Work out the finished part from the listing and answer in its coordinate system (mm). Face numbers are marked on the shaded views. A direction names the side the tool comes from. Coordinates: 2 decimals unless noted, no trailing zeros. Order: outer loops, then holes, each group sorted by start corner. A loop starts at its lowest first (then second) coordinate and runs counter-clockwise, first axis right, second up. Notation, with made-up numbers: M 47,85 L 67,85 A26 cw 67,115 Z; hole C -20.75,16 d3. An arc over 180 degrees is marked long. Write item = value, one per line. Start each with the question number.
Q1. Each of these flat-tipped pins is pushed along its axis until it touches: P1, Ø6, axis at x = -9.5, y = -1.5, coming from the +Z side; P2, Ø12, axis at x = -5, y = -5, coming from the -Z side; P3, Ø4.5, axis at x = 3.75, y = 0, coming from the +Z side; P4, Ø4, axis at x = -3.75, y = 0, coming from the +Z side. Where does it stop, or does it pass through?
Q2. Straight lines are drawn through the part: line 1 along Y through (x, z) = (-25, 1.55); line 2 along Y through (x, z) = (-14.5, 6.25); line 3 along Z through (x, y) = (-6.5, 3.75). For each, find the intervals that lie inside material, in ascending order.
Q3. Find section C-C on z = 3.5. Give the vertices of the cut face in (x, y).
Q4. A tool of negligible diameter and unlimited length cuts with its end or side. For the marked faces 4 and 5, from which of +Z, -Z, +X, -X, +Y, -Y can it reach the whole face along a straight path? Write none if from no direction.
Q5. Determine the mould class of the marked faces 1, 2 and 3 for opening direction Y: released by +Y, released by -Y, zero draft, split by the parting line, or undercut.
Q6. Find section A-A on y = 0. Give the vertices of the cut face in (x, z).
Q7. Find section D-D on x = 15. Give the vertices of the cut face in (y, z).
Q8. Find section B-B on x = -3.75. Give the vertices of the cut face in (y, z).
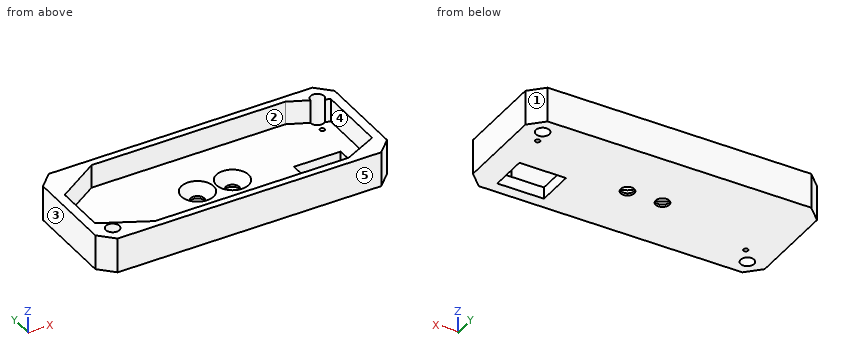
```python
from build123d import *

# Parameters (mm, degrees)
SKETCH_1_W          = 62.5
SKETCH_1_H          = 25
EXTRUDE_1_DEPTH     = 2.5
SKETCH_2_R          = 1.45
CUT_EXTRUDE_1_DEPTH = 3.5
CHAMFER_1_SIZE      = 2
SKETCH_3_W          = 62.5
SKETCH_3_H          = 25
EXTRUDE_2_DEPTH     = 5
SKETCH_4_W          = 10
SKETCH_4_H          = 8
CUT_EXTRUDE_2_DEPTH = 5
SKETCH_5_W          = 67.566121691
SKETCH_5_H          = 29.988395665
CUT_EXTRUDE_3_DEPTH = 10
SKETCH_7_R          = 1.45
CUT_EXTRUDE_4_DEPTH = 10
SKETCH_10_R         = 0.5
CUT_EXTRUDE_5_DEPTH = 10


with BuildPart() as part:
    # Эскиз1 → Бобышка-Вытянуть1 (new body)
    with BuildSketch(Plane.XY):
        Rectangle(SKETCH_1_W, SKETCH_1_H)
    extrude(amount=EXTRUDE_1_DEPTH)

    # Эскиз2 → Вырез-Вытянуть1 (cut)
    with BuildSketch(Plane.XY.offset(2.5)):
        with Locations((3.75, 0)):
            Circle(SKETCH_2_R)
        with Locations((-3.75, 0)):
            Circle(SKETCH_2_R)
    extrude(amount=-CUT_EXTRUDE_1_DEPTH, mode=Mode.SUBTRACT)

    # Фаска1
    chamfer_1_edges = [part.edges().sort_by_distance(p)[0] for p in [
        (2.3, 0, 2.5),
        (-5.2, 0, 2.5),
    ]]
    chamfer(chamfer_1_edges, length=CHAMFER_1_SIZE)

    # Эскиз3 → Бобышка-Вытянуть2 (add)
    with BuildSketch(Plane.XY.offset(2.5)):
        Rectangle(SKETCH_3_W, SKETCH_3_H)
        Polygon((-29.25, -6), (-29.25, 5), (-19.95, 11), (21.55, 11), (29.25, 7.5), (29.25, -7.5), (22.14795897, -11), (-19.35204103, -11), align=None, mode=Mode.SUBTRACT)
    extrude(amount=EXTRUDE_2_DEPTH)

    # Эскиз4 → Вырез-Вытянуть2 (cut)
    with BuildSketch(Plane(origin=(0, 0, 0), x_dir=(-1, 0, 0), z_dir=(0, 0, -1))):
        with Locations((-20.75, -6)):
            Rectangle(SKETCH_4_W, SKETCH_4_H)
    extrude(amount=-CUT_EXTRUDE_2_DEPTH, mode=Mode.SUBTRACT)

    # Эскиз5 → Вырез-Вытянуть3 (cut)
    with BuildSketch(Plane.XY.offset(7.5)):
        with Locations((0.466014855, 0.289583976)):
            Rectangle(SKETCH_5_W, SKETCH_5_H)
        Polygon((-28.25, 12.5), (-31.25, 9.5), (-31.25, -9.5), (-28.25, -12.5), (28.25, -12.5), (31.25, -9.5), (31.25, 9.5), (28.25, 12.5), align=None, mode=Mode.SUBTRACT)
    extrude(amount=-CUT_EXTRUDE_3_DEPTH, mode=Mode.SUBTRACT)

    # Эскиз7 → Вырез-Вытянуть4 (cut)
    with BuildSketch(Plane.XY.offset(7.5)):
        with Locations((-27.25, -9)):
            Circle(SKETCH_7_R)
        with Locations(Location((27.25, 9, 0), (0, 0, 313.779004768))):
            Circle(SKETCH_7_R)
    extrude(amount=-CUT_EXTRUDE_4_DEPTH, mode=Mode.SUBTRACT)

    # Эскиз10 → Вырез-Вытянуть5 (cut)
    with BuildSketch(Plane.XY.offset(2.5)):
        with Locations((-25, -5.766085635)):
            Circle(SKETCH_10_R)
        with Locations((26.547958971, 6)):
            Circle(SKETCH_10_R)
    extrude(amount=-CUT_EXTRUDE_5_DEPTH, mode=Mode.SUBTRACT)


solid = part.part
```
Findings below:
q1.P1 = 2.5
q1.P2 = 0
q1.P3 = 1.3
q1.P4 = 1.05
q2.line_1 = -12.5 to -6.27, -5.27 to 12.5
q2.line_2 = -12.5 to -11, 11 to 12.5
q2.line_3 = 0 to 2.5
q3.outline = M -31.25,-9.5 L -28.25,-12.5 L 28.25,-12.5 L 31.25,-9.5 L 31.25,9.5 L 28.25,12.5 L -28.25,12.5 L -31.25,9.5 Z; hole M -29.25,-6 L -19.35,-11 L 22.15,-11 L 24.18,-10 L 25.75,-10 L 25.75,-9.22 L 29.25,-7.5 L 29.25,7.5 L 28.25,7.95 A1.45 ccw long 25.8,9.07 L 21.55,11 L -19.95,11 L -29.25,5 Z; hole C -27.25,-9 d2.9
q4.face_4 = +Z
q4.face_5 = +Z, -Z, +X, -X, -Y
q5.face_1 = released by +Y
q5.face_2 = undercut
q5.face_3 = zero draft
q6.outline = M -31.25,0 L -5.2,0 L -5.2,0.5 L -7.2,2.5 L -29.25,2.5 L -29.25,7.5 L -31.25,7.5 Z; M -2.3,0 L 2.3,0 L 2.3,0.5 L 0.3,2.5 L -0.3,2.5 L -2.3,0.5 Z; M 5.2,0 L 31.25,0 L 31.25,7.5 L 29.25,7.5 L 29.25,2.5 L 7.2,2.5 L 5.2,0.5 Z
q7.outline = M -12.5,0 L 12.5,0 L 12.5,7.5 L 11,7.5 L 11,2.5 L -11,2.5 L -11,7.5 L -12.5,7.5 Z
q8.outline = M -12.5,0 L -1.45,0 L -1.45,0.5 L -3.45,2.5 L -11,2.5 L -11,7.5 L -12.5,7.5 Z; M 1.45,0 L 12.5,0 L 12.5,7.5 L 11,7.5 L 11,2.5 L 3.45,2.5 L 1.45,0.5 Z
